Work out the finished part from the listing and answer in its coordinate system (mm). A direction names the side the tool comes from. Give positions to 0.01 mm unless a question says otherwise; leave off trailing zeros. Loops run counter-clockwise (first coordinate to the right, second up) from the corner with the lowest first, then second, coordinate; pieces in that order, holes last. Notation, with made-up numbers: M -14,79 L 39,79 A22 cw 39,96 Z; hole C -33.5,22.5 d10. An arc over 180 degrees is marked long. Use a Markdown table: item, result.
```python
from build123d import *

# Parameters (mm, degrees)
F0_W     = 1.5875
F0_H     = 12.3
F1_DEPTH = 3.175


# Not quite as in the source:
# - a length typed as a fraction of an inch, garbled in the dataset ("3 / 203.2 mm" for 3/8 in), is restored
# - a feature names something its author has since deleted; it is built from what else it names


with BuildPart() as f1:
    # F0 (on Front) → F1 (new body)
    with BuildSketch(Plane.XZ):
        with Locations((21.70625, 0)):
            Rectangle(F0_W, F0_H)
        with Locations((-21.70625, 0)):
            Rectangle(F0_W, F0_H)
        Polygon((-22.5, -16.15), (-22.5, -22.5), (-16.15, -22.5), (-16.15, -25.675), (-6.15, -25.675), (-6.15, -22.5), (6.15, -22.5), (6.15, -25.675), (16.15, -25.675), (16.15, -22.5), (22.5, -22.5), (22.5, -16.15), (19.325, -16.15), (19.325, -6.15), (20.9125, -6.15), (20.9125, 6.15), (19.325, 6.15), (19.325, 16.15), (16.15, 16.15), (16.15, 19.325), (6.15, 19.325), (6.15, 16.15), (-6.15, 16.15), (-6.15, 19.325), (-16.15, 19.325), (-16.15, 16.15), (-19.325, 16.15), (-19.325, 6.15), (-20.9125, 6.15), (-20.9125, -6.15), (-19.325, -6.15), (-19.325, -16.15), align=None)
    extrude(amount=F1_DEPTH)


solid = f1.part
```
(1) The mould has two halves that part along X. Classify faces 1 (the flat face through (-21, -2, -16.15)), 2 (the flat face through (0, -2, -22.5)), 3 (the flat face through (22.5, -2, -19)): released by +X, released by -X, zero draft, split by the parting line, or undercut.
Entries:
| item | result |
|---|---|
| face 1 | zero draft |
| face 2 | undercut |
| face 3 | released by +X |
(2) Which of the six approach directions +Z, -Z, +X, -X, +Y, -Y give full straight-line access (tool end or side, diameter ignored) to faces 4 (the flat face through (-6.15, -2, -24)), 5 (the flat face through (-18, -2, 16.15)), 6 (the flat face through (19.325, -2, 11)), 7 (the flat face through (19.325, -2, -11))?
Entries:
| item | result |
|---|---|
| face 4 | -Z, +Y, -Y |
| face 5 | +Z, -X, +Y, -Y |
| face 6 | +Z, +X, +Y, -Y |
| face 7 | +X, +Y, -Y |
(3) A cutting plane is placed at C-C (z = 15.5). Write down the section's boundary in (x, y) (3 decimals), and give its area (3 significant figures).
Entries:
| item | result |
|---|---|
| outline | M -19.325,-3.175 L 19.325,-3.175 L 19.325,0 L -19.325,0 Z |
| area | 123 mm² |
(4) A cutting plane is placed at B-B (x = -2). Write down the section's boundary in (y, z) (3 decimals), and give its area (3 significant figures).
Entries:
| item | result |
|---|---|
| outline | M -3.175,-22.5 L 0,-22.5 L 0,16.15 L -3.175,16.15 Z |
| area | 123 mm² |
(5) Consider probe 1 along Z at (x, y) = (21.5, -0.2); probe 2 along X at (y, z) = (-1.15, 16.5); probe 3 along X at (y, z) = (-0.5, -13) (3 decimals). Determine where each line is inside the solid, lowest interval first. Write a range as [from, to].
Entries:
| item | result |
|---|---|
| probe 1 | z = [-22.5, -16.15], [-6.15, 6.15] |
| probe 2 | x = [-16.15, -6.15], [6.15, 16.15] |
| probe 3 | x = [-19.325, 19.325] |
(6) Given P1, Ø1.6, axis at y = -1.5, z = 18.5, coming from the -X side; P2, Ø1, axis at x = -2, y = -1, coming from the +Z side; P3, Ø1, axis at y = -1.5, z = -12, coming from the +X side (3 decimals), each flat-ended and moving along its own axis, determine where each tip first touches the part or whether it passes through.
Entries:
| item | result |
|---|---|
| P1 | stops at x = -16.15 |
| P2 | stops at z = 16.15 |
| P3 | stops at x = 19.325 |
